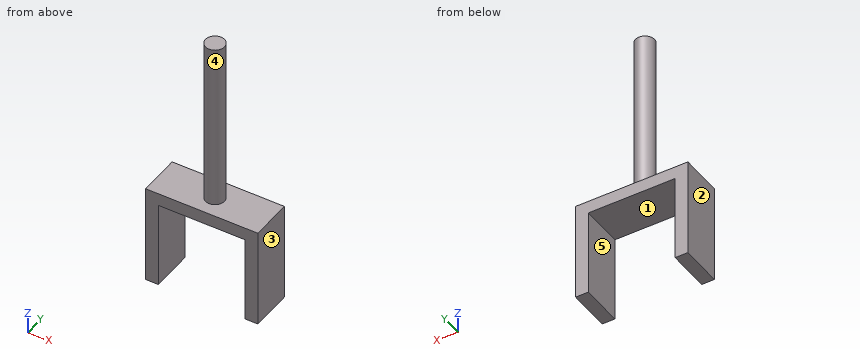
from build123d import *

# Parameters (mm, degrees)
F0_W     = 20.5
F0_H     = 3
F1_DEPTH = 10
F2_R     = 2.25
F3_DEPTH = 40


with BuildPart() as f1:
    # F0 (on Front) → F1 (new body)
    with BuildSketch(Plane.XZ):
        Polygon((-17.136792, -6.331904), (-14.136792, -6.331904), (-14.136792, 14.168096), (-14.136792, 17.168096), (-17.136792, 17.168096), align=None)
        with Locations((-3.886792, 15.668096)):
            Rectangle(F0_W, F0_H)
        Polygon((6.363208, 14.168096), (6.363208, -6.331904), (9.363208, -6.331904), (9.363208, 17.168096), (6.363208, 17.168096), align=None)
    extrude(amount=F1_DEPTH)

    # F2 (on face) → F3 (join)
    with BuildSketch(Plane.XY.offset(17.168096)):
        with Locations((-3.886792, -5)):
            Circle(F2_R)
    extrude(amount=F3_DEPTH)


solid = f1.part
Could you check a few things on this model? Use its own coordinates, in mm. Face numbers are marked on the shaded views. A direction names the side the tool comes from. Give positions to 0.01 mm unless a question says otherwise; leave off trailing zeros. Order: outer loops, then holes, each group sorted by start corner. A loop starts at its lowest first (then second) coordinate and runs counter-clockwise, first axis right, second up. Notation, with made-up numbers: (1.25, 85) -> (25.25, 85) arc R23 ccw to (25.25, 96) -> close; hole circle Ø3 at (8, 55). An arc over 180 degrees is marked (long way). Answer in a Markdown table with one row per item. Add a question column.
Item 1: Imagine slicing it at A-A (y = -1.5). List the corners of the cut face in (x, z) for me.
Item 2: For the marked faces 1 and 2, which set-ups out of +Z, -Z, +X, -X, +Y, -Y let a thin tool reach every point of the face, with its end or its side?
Item 3: I'm going to push flat-ended pins straight in: P1, Ø6, axis at x = -4.5, z = 31.5, coming from the +Y side; P2, Ø1.5, axis at x = 3.5, y = -8.5, coming from the -Z side; P3, Ø5, axis at y = -8.5, z = 44, coming from the -X side. Where does each tip first touch, or does it pass through?
Item 4: Please list where these lines run through material, in increasing order: probe 1 along X at (y, z) = (-1.5, 9); probe 2 along Z at (x, y) = (-10, -0.25); probe 3 along Z at (x, y) = (7.75, -0.5).
Item 5: Imagine slicing it at D-D (y = -5). List the corners of the cut face in (x, z) for me.
Item 6: Imagine slicing it at B-B (x = -3). List the corners of the cut face in (y, z) for me, and give its area (3 significant figures).
Item 7: Imagine slicing it at C-C (z = 37.5). List the corners of the cut face in (x, y) for me.
Item 8: We'd pull the mould along X, two halves only. Please class the marked faces 3, 4 and 5: pulls with the +X half, pulls with the -X half, needs draft (parallel to the pull), parting line crosses it, or undercut.
Result:
| question | item | result |
|---|---|---|
| 1 | outline | (-17.14, -6.33) -> (-14.14, -6.33) -> (-14.14, 14.17) -> (6.36, 14.17) -> (6.36, -6.33) -> (9.36, -6.33) -> (9.36, 17.17) -> (-17.14, 17.17) -> close |
| 2 | face 1 | -Z, +Y, -Y |
| 2 | face 2 | +Z, -Z, -X, +Y, -Y |
| 3 | P1 | y = -2.75 |
| 3 | P2 | z = 14.17 |
| 3 | P3 | x = -5.9 |
| 4 | probe 1 | -17.14 to -14.14, 6.36 to 9.36 |
| 4 | probe 2 | 14.17 to 17.17 |
| 4 | probe 3 | -6.33 to 17.17 |
| 5 | outline | (-17.14, -6.33) -> (-14.14, -6.33) -> (-14.14, 14.17) -> (6.36, 14.17) -> (6.36, -6.33) -> (9.36, -6.33) -> (9.36, 17.17) -> (-1.64, 17.17) -> (-1.64, 57.17) -> (-6.14, 57.17) -> (-6.14, 17.17) -> (-17.14, 17.17) -> close |
| 6 | outline | (-10, 14.17) -> (0, 14.17) -> (0, 17.17) -> (-2.93, 17.17) -> (-2.93, 57.17) -> (-7.07, 57.17) -> (-7.07, 17.17) -> (-10, 17.17) -> close |
| 6 | area | 195 mm2 |
| 7 | outline | circle Ø4.5 at (-3.89, -5) |
| 8 | face 3 | pulls with the +X half |
| 8 | face 4 | parting line crosses it |
| 8 | face 5 | undercut |
